Read the model definition and answer for the solid it produces. Units are mm, in the model's axes. A direction names the side the tool comes from. Coordinates: 2 decimals unless noted, no trailing zeros. Write each loop counter-clockwise with the first axis right and the second up, starting at its lowest first coordinate (ties: lowest second). Pieces come first, ordered by that corner, then holes. Notation, with made-up numbers: (88.5, -25) -> (136.5, -25) arc R24 ccw to (136.5, -14) -> close; hole circle Ø6 at (0, 33). An arc over 180 degrees is marked (long way). One line per item, written item: value. Start each with the question number.
from build123d import *

# Parameters (mm, degrees)
SKETCH1_R           = 13.25
BOSS_EXTRUDE1_DEPTH = 35
SKETCH7_R           = 10
CUT_EXTRUDE4_DEPTH  = 8
SKETCH10_R          = 3.485
BOSS_EXTRUDE3_DEPTH = 4
SKETCH11_R          = 1.625
CUT_EXTRUDE5_DEPTH  = 8.75
SKETCH13_R          = 10
CUT_EXTRUDE6_DEPTH  = 18


with BuildPart() as part:
    # Sketch1 → Boss-Extrude1 (new body)
    with BuildSketch(Plane(origin=(0, 0, 0), x_dir=(1, 0, 0), z_dir=(0, 1, 0))):
        Circle(SKETCH1_R)
    extrude(amount=BOSS_EXTRUDE1_DEPTH)

    # Sketch7 → Cut-Extrude4 (cut)
    with BuildSketch(Plane.XZ):
        Circle(SKETCH7_R)
    extrude(amount=-CUT_EXTRUDE4_DEPTH, mode=Mode.SUBTRACT)

    # Sketch10 → Boss-Extrude3 (add)
    with BuildSketch(Plane.XZ.offset(-8)):
        Circle(SKETCH10_R)
    extrude(amount=BOSS_EXTRUDE3_DEPTH)

    # Sketch11 → Cut-Extrude5 (cut)
    with BuildSketch(Plane.XZ.offset(-4)):
        Circle(SKETCH11_R)
    extrude(amount=-CUT_EXTRUDE5_DEPTH, mode=Mode.SUBTRACT)

    # Sketch13 → Cut-Extrude6 (cut)
    with BuildSketch(Plane(origin=(0, 35, 0), x_dir=(1, 0, 0), z_dir=(0, 1, 0))):
        Circle(SKETCH13_R)
    extrude(amount=-CUT_EXTRUDE6_DEPTH, mode=Mode.SUBTRACT)


solid = part.part
1. For a pull along X with two mould halves and no side action, classify faces 1 (the face through (2, 35, -10)), 2 (the face through (2, 4, -1)), 3 (the face through (7.123, 17.255, -11.172)) as +X half, -X half, draft (parallel to the pull), parting line (faces both ways), or undercut.
2. A cutting plane is placed at A-A on y = 6.5. Give the vertices of the cut face in (x, z) (3 decimals), then the cut area to 3 significant figures.
3. Given pin 1 (6 mm diameter, centred on x = -4, z = -4.5, fed in from -Y); pin 2 (5 mm diameter, centred on x = -7.5, y = 24, fed in from -Z); pin 3 (2 mm diameter, centred on x = 4, z = 7.5, fed in from +Y), each flat-ended and moving along its own axis, determine where each tip first touches the part or whether it passes through.
4. A cutting plane is placed at B-B on z = 0. Give the vertices of the cut face in (x, y) (3 decimals).
5. A cutting plane is placed at C-C on x = 0. Give the vertices of the cut face in (y, z) (3 decimals).
6. A cutting plane is placed at D-D on y = 31. Give the vertices of the cut face in (x, z), then the cut area to 3 significant figures.
7. Find the intervals of material crossed by probe 1 along Z at (x, y) = (0, 21.5); probe 2 along Z at (x, y) = (0, 10) (3 decimals); probe 3 along Y at (x, z) = (6, 2.25), in increasing order. Write a range as from..to.
8. A tool of negligible diameter and unlimited length cuts with its end or side. For faces 4 (the face through (2, 0, -10)), 5 (the face through (0, 12.75, 0)), 6 (the face through (0, 17, 0)), from which of +Z, -Z, +X, -X, +Y, -Y can it reach the whole face along a straight path? Write none if from no direction.
Derived:
1. face 1: draft
1. face 2: undercut
1. face 3: parting line
2. outline: circle Ø26.5 at (0, 0); circle Ø6.97 at (0, 0); hole circle Ø20 at (0, 0); hole circle Ø3.25 at (0, 0)
2. area: 267 mm2
3. pin 1: stops at y = 4
3. pin 2: stops at z = -12.27
3. pin 3: stops at y = 17
4. outline: (-13.25, 0) -> (-10, 0) -> (-10, 8) -> (-3.485, 8) -> (-3.485, 4) -> (-1.625, 4) -> (-1.625, 12.75) -> (1.625, 12.75) -> (1.625, 4) -> (3.485, 4) -> (3.485, 8) -> (10, 8) -> (10, 0) -> (13.25, 0) -> (13.25, 35) -> (10, 35) -> (10, 17) -> (-10, 17) -> (-10, 35) -> (-13.25, 35) -> close
5. outline: (0, -13.25) -> (35, -13.25) -> (35, -10) -> (17, -10) -> (17, 10) -> (35, 10) -> (35, 13.25) -> (0, 13.25) -> (0, 10) -> (8, 10) -> (8, 3.485) -> (4, 3.485) -> (4, 1.625) -> (12.75, 1.625) -> (12.75, -1.625) -> (4, -1.625) -> (4, -3.485) -> (8, -3.485) -> (8, -10) -> (0, -10) -> close
6. outline: circle Ø26.5 at (0, 0); hole circle Ø20 at (0, 0)
6. area: 237 mm2
7. probe 1: z = -13.25..-10, 10..13.25
7. probe 2: z = -13.25..-1.625, 1.625..13.25
7. probe 3: y = 8..17
8. face 4: +Z, -Z, +X, -X, -Y
8. face 5: -Y
8. face 6: +Y
